Verification items for the finished model (mm, model axes). A direction names the side the tool comes from. Coordinates: 2 decimals unless noted, no trailing zeros. Order: outer loops, then holes, each group sorted by start corner. A loop starts at its lowest first (then second) coordinate and runs counter-clockwise, first axis right, second up. Notation, with made-up numbers: (35, 57.25) -> (84, 57.25) arc R33 ccw to (84, 88.25) -> close; hole circle Ø4 at (3, -3). An arc over 180 degrees is marked (long way). Write item = value, one per line. Start each with the question number.
1. Cross-section at B-B on x = -10. Record the cut outline in (y, z).
2. Set-up check for faces 4 (the flat face through (21, 68.3, -35)), 5 (the cylindrical face through (41.593, 20.967, -3.479)): record each of +Z, -Z, +X, -X, +Y, -Y from which the full face is reachable in a straight line by a thin tool's end or side.
3. Thickness scan on line 1 along Y through (x, z) = (22.5, -3.25); line 2 along Y through (x, z) = (31.3, -4); line 3 along X through (y, z) = (52, -8.5). Record the ranges inside material, lowest first. Write a range as from..to.
4. Go/stop test with flat-tipped pins: P1, Ø3, axis at x = 17.5, y = 57.5, coming from the +Z side; P2, Ø3, axis at x = 33, y = 25.5, coming from the -Z side; P3, Ø1.3, axis at x = 42.5, y = 23.5, coming from the -Z side. Record where each tip stops, or that it passes through.
5. Cross-section at C-C on y = 56. Record the cut outline in (x, z).
6. Cross-section at D-D on y = 6.3. Record the cut outline in (x, z).
7. Release check for a two-part mould opening along X. For faces 1 (the flat face through (61.8, 25, -35)), 2 (the flat face through (21, -18, -35)), 3 (the flat face through (5, 39, -5)) record: +X half, -X half, draft (parallel to the pull), parting line (faces both ways), or undercut.
8. Cross-section at A-A on z = -28.5. Record the cut outline in (x, y).
from build123d import *

# Parameters (mm, degrees)
F1_W     = 79.8
F1_H     = 86.3
F1_W_2   = 75.8
F1_H_2   = 82.3
F2_DEPTH = 70
F3_DEPTH = 2
F4_R     = 3.35
F4_R_2   = 1.35
F4_R_3   = 2.8
F4_R_4   = 0.8
F5_DEPTH = 5


with BuildPart() as f2:
    # F1 (on Top) → F2 (new body)
    with BuildSketch(Plane.XY):
        with Locations((21.9, 25.15)):
            Rectangle(F1_W, F1_H)
        with Locations((21.9, 25.15)):
            Rectangle(F1_W_2, F1_H_2, mode=Mode.SUBTRACT)
    extrude(amount=-F2_DEPTH)

    # F1 (on Top) → F3 (join)
    with BuildSketch(Plane.XY):
        with Locations((21.9, 25.15)):
            Rectangle(F1_W_2, F1_H_2)
    extrude(amount=-F3_DEPTH)

    # F4 (on Top) → F5 (join)
    with BuildSketch(Plane.XY):
        with Locations((22.5, 6.3)):
            Circle(F4_R)
        with Locations((22.5, 6.3)):
            Circle(F4_R_2, mode=Mode.SUBTRACT)
        with Locations((42.2, 23.7)):
            Circle(F4_R_3)
        with Locations((42.2, 23.7)):
            Circle(F4_R_4, mode=Mode.SUBTRACT)
        with Locations((22.4, 29.5)):
            Circle(F4_R_3)
        with Locations((22.4, 29.5)):
            Circle(F4_R_4, mode=Mode.SUBTRACT)
        with Locations((4.2, 40)):
            Circle(F4_R_3)
        with Locations((4.2, 40)):
            Circle(F4_R_4, mode=Mode.SUBTRACT)
        with Locations((43.8, 42.1)):
            Circle(F4_R_3)
        with Locations((43.8, 42.1)):
            Circle(F4_R_4, mode=Mode.SUBTRACT)
        with Locations((31.3, 50.3)):
            Circle(F4_R_3)
        with Locations((31.3, 50.3)):
            Circle(F4_R_4, mode=Mode.SUBTRACT)
    extrude(amount=-F5_DEPTH)


solid = f2.part
Worked out:
q1.outline = (-18, -70) -> (-16, -70) -> (-16, -2) -> (66.3, -2) -> (66.3, -70) -> (68.3, -70) -> (68.3, 0) -> (-18, 0) -> close
q2.face_4 = +Z, -Z, +X, -X, +Y
q2.face_5 = -Z
q3.line_1 = -18..-16, 2.95..4.95, 7.65..9.65, 26.7..28.71, 30.29..32.3, 66.3..68.3
q3.line_2 = -18..-16, 47.5..49.5, 51.1..53.1, 66.3..68.3
q3.line_3 = -18..-16, 59.8..61.8
q4.P1 = 0
q4.P2 = -2
q4.P3 = -5
q5.outline = (-18, -70) -> (-16, -70) -> (-16, -2) -> (59.8, -2) -> (59.8, -70) -> (61.8, -70) -> (61.8, 0) -> (-18, 0) -> close
q6.outline = (-18, -70) -> (-16, -70) -> (-16, -2) -> (19.15, -2) -> (19.15, -5) -> (21.15, -5) -> (21.15, -2) -> (23.85, -2) -> (23.85, -5) -> (25.85, -5) -> (25.85, -2) -> (59.8, -2) -> (59.8, -70) -> (61.8, -70) -> (61.8, 0) -> (-18, 0) -> close
q7.face_1 = +X half
q7.face_2 = draft
q7.face_3 = undercut
q8.outline = (-18, -18) -> (61.8, -18) -> (61.8, 68.3) -> (-18, 68.3) -> close; hole (-16, -16) -> (59.8, -16) -> (59.8, 66.3) -> (-16, 66.3) -> close
